from build123d import *

# Parameters (mm, degrees)
F0_R      = 4.25
F1_DEPTH  = 5
F3_DEPTH  = 2
F4_R      = 2.5
F5_DEPTH  = 40
F5_FACE_R = 2.5
F6_DEPTH  = 22.7
F7_DEPTH  = 21.3


with BuildPart() as f1:
    # F0 (on Top) → F1 (new body)
    with BuildSketch(Plane.XY):
        Circle(F0_R)
    extrude(amount=F1_DEPTH)

    # F2 (on face) → F3 (cut)
    with BuildSketch(Plane.XY.offset(5)):
        Polygon((2, -1.154701), (2, 1.154701), (0, 2.309401), (-2, 1.154701), (-2, -1.154701), (0, -2.309401), align=None)
    extrude(amount=-F3_DEPTH, mode=Mode.SUBTRACT)

    # F4 (on Top) → F5 (join)
    with BuildSketch(Plane.XY):
        Circle(F4_R)
    extrude(amount=-F5_DEPTH)

    # F5_face (on face) → F6 (join)
    with BuildSketch(Plane(origin=(0, 0, -40), x_dir=(1, 0, 0), z_dir=(0, 0, -1))):
        Circle(F5_FACE_R)
    extrude(amount=-F6_DEPTH)

    # F5_face (on face) → F7 (cut)
    with BuildSketch(Plane(origin=(0, 0, -40), x_dir=(1, 0, 0), z_dir=(0, 0, -1))):
        Circle(F5_FACE_R)
    extrude(amount=-F7_DEPTH, mode=Mode.SUBTRACT)


solid = f1.part
Work out the finished part from the listing and answer in its coordinate system (mm). A direction names the side the tool comes from. Round coordinates to 2 decimals unless told otherwise and drop trailing zeros. Write each loop counter-clockwise with the first axis right and the second up, starting at its lowest first coordinate (ties: lowest second). Pieces come first, ordered by that corner, then holes.
1) A cutting plane is placed at A-A (z = 3.75). Give the vertices of the cut face in (x, y).
2) A tool of negligible diameter and unlimited length cuts with its end or side. For faces 1 (the flat face through (2, -2, 0)), 2 (the flat face through (0, 0, -18.7)), 3 (the flat face through (0, 0, 3)), from which of +Z, -Z, +X, -X, +Y, -Y can it reach the whole face along a straight path? Write none if from no direction.
3) Straight lines are drawn through the part: line 1 (X direction, y = -1.5, z = -10); line 2 (Z direction, x = -0.5, y = 3.75). For each, find the intervals that lie inside material, in ascending order.
4) Given pin 1 Ø1 at (x, y) = (0.5, 3) entering from -Z; pin 2 Ø5 at (x, z) = (-1, -13.5) entering from -Y; pin 3 Ø1 at (y, z) = (-1.5, 1) entering from +X, each flat-ended and moving along its own axis, determine where each tip first touches the part or whether it passes through.
5) A cutting plane is placed at D-D (x = 3.5). Give the vertices of the cut face in (y, z), plus the area to 3 significant figures.
6) A cutting plane is placed at B-B (y = 0). Give the vertices of the cut face in (x, z).
7) A cutting plane is placed at C-C (z = -0.25). Give the vertices of the cut face in (x, y), plus the area to 3 significant figures.
8) The mould has two halves that part along Y. Classify faces 4 (the flat face through (1, -2, 5)), 5 (the cylindrical face through (-0.54, -2.44, -9.22)), 6 (the flat face through (-0.99, 1.74, 4.01)): pulls with the +Y half, pulls with the -Y half, needs draft (parallel to the pull), parting line crosses it, or undercut.
Completed:
1. outline: circle Ø8.5 at (0, 0); hole (-2, -1.15) - (0, -2.31) - (2, -1.15) - (2, 1.15) - (0, 2.31) - (-2, 1.15) - close
2. face 1: -Z
2. face 2: -Z, +X, -X, +Y, -Y
2. face 3: +Z
3. line 1: x = -2 to 2
3. line 2: z = 0 to 5
4. pin 1: stops at z = 0
4. pin 2: stops at y = -2.5
4. pin 3: stops at x = 4.13
5. outline: (-2.41, 0) - (2.41, 0) - (2.41, 5) - (-2.41, 5) - close
5. area: 24.1 mm2
6. outline: (-4.25, 0) - (-2.5, 0) - (-2.5, -18.7) - (2.5, -18.7) - (2.5, 0) - (4.25, 0) - (4.25, 5) - (2, 5) - (2, 3) - (-2, 3) - (-2, 5) - (-4.25, 5) - close
7. outline: circle Ø5 at (0, 0)
7. area: 19.6 mm2
8. face 4: needs draft
8. face 5: parting line crosses it
8. face 6: undercut
